For this review, use the dimensioned drawing (mm, ordinates from the lowest corner) and the shaded views. Give positions to 0.01 mm unless a question says otherwise; leave off trailing zeros. Write each loop counter-clockwise with the first axis right and the second up, starting at its lowest first coordinate (ties: lowest second). Pieces come first, ordered by that corner, then holes. Notation, with made-up numbers: M 16.25,-16 L 67.25,-16 A28 ccw 67.25,11 Z; hole C 28.5,9.25 d1. An arc over 180 degrees is marked long. Use a Markdown table: item, result. Add a question column.
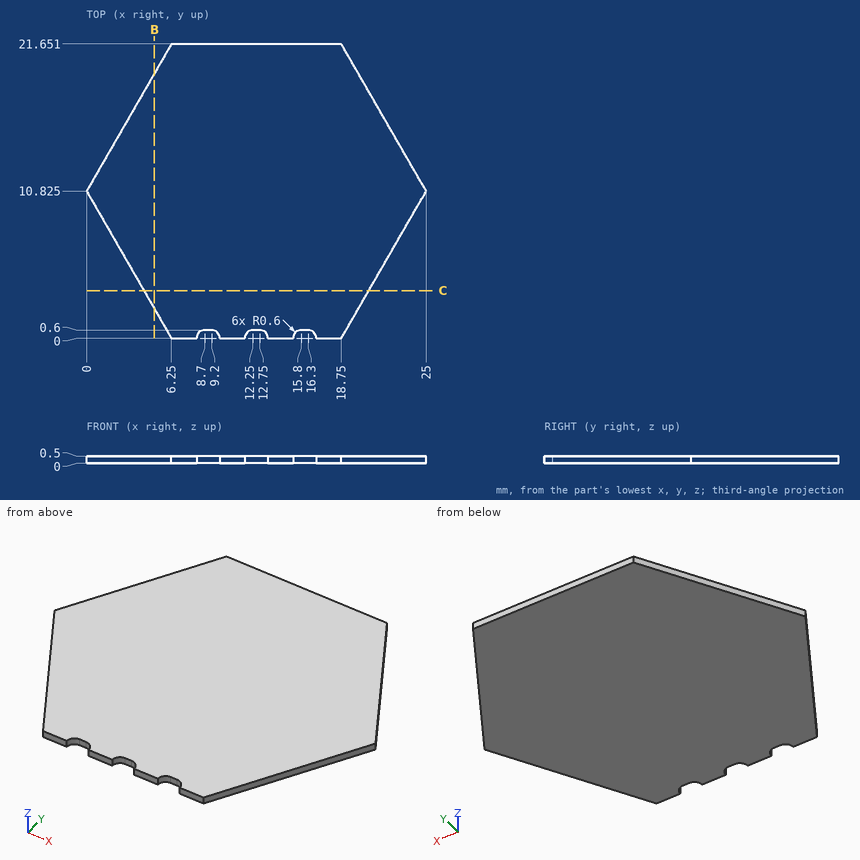
(1) Add section B-B on x = 5. Give the boundary of the cut face in (y, z) (1 decimal).
(2) Wall thickness on L1, parallel to Y at x = 12.25, z = 0.35; L2, parallel to Y at x = 19.5, z = 0.4; L3, parallel to X at y = 20.5, z = 0.4 (1 decimal): over which ranges is each line inside the solid? List them lowest first.
(3) Add section C-C on y = 3.5. Give the boundary of the cut face in (x, z).
From the geometry:
| question | item | result |
|---|---|---|
| 1 | outline | M 2.2,0 L 19.5,0 L 19.5,0.5 L 2.2,0.5 Z |
| 2 | L1 | y = 0.6 to 21.65 |
| 2 | L2 | y = 1.3 to 20.35 |
| 2 | L3 | x = 5.6 to 19.4 |
| 3 | outline | M 4.23,0 L 20.77,0 L 20.77,0.5 L 4.23,0.5 Z |
